Geometry check sheet. Reference: the model listing, model coordinates, mm. Coordinates: 2 decimals unless noted, no trailing zeros. Write each loop counter-clockwise with the first axis right and the second up, starting at its lowest first coordinate (ties: lowest second). Pieces come first, ordered by that corner, then holes. Notation, with made-up numbers: M 13,-21.75 L 35,-21.75 A12 cw 35,-8.75 Z; hole C 80.25,-15.75 d4. An arc over 180 degrees is marked long. Answer as a JSON object with one key per item and string values. Group by question number.
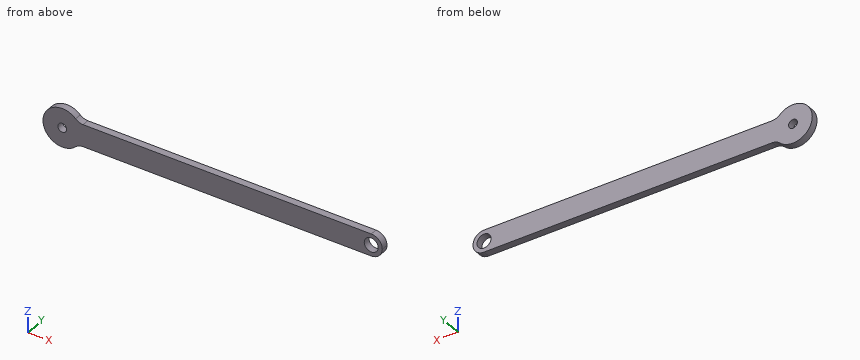
```python
from build123d import *

# Parameters (mm, degrees)
SKETCH1_W           = 300
SKETCH1_H           = 20
BOSS_EXTRUDE1_DEPTH = 6.35
SKETCH2_R           = 6.35
CUT_EXTRUDE1_DEPTH  = 6.35
CONG_1_R            = 10
SKETCH3_R           = 17.5
SKETCH3_R_2         = 4
BOSS_EXTRUDE2_DEPTH = 6.35
FILLET2_R           = 10


with BuildPart() as part:
    # Sketch1 → Boss-Extrude1 (new body)
    with BuildSketch(Plane(origin=(0, 0, 0), x_dir=(1, 0, 0), z_dir=(0, 1, 0))):
        Rectangle(SKETCH1_W, SKETCH1_H)
    extrude(amount=BOSS_EXTRUDE1_DEPTH)

    # Sketch2 → Cut-Extrude1 (cut)
    with BuildSketch(Plane(origin=(0, 0, 0), x_dir=(-1, 0, 0), z_dir=(0, -1, 0))):
        with Locations(Location((140, 0, 0), (0, 0, 90))):
            Circle(SKETCH2_R)
    cut_extrude1 = extrude(amount=-CUT_EXTRUDE1_DEPTH, mode=Mode.SUBTRACT)

    # Mirror1: Cut-Extrude1 across plane
    add(cut_extrude1.mirror(Plane(origin=(0, 0, 0), x_dir=(0, 0, 1), z_dir=(1, 0, 0))), mode=Mode.SUBTRACT)

    # Congé1
    cong_1_edges = [part.edges().sort_by_distance(p)[0] for p in [
        (-150, 3.175, -10),
        (-150, 3.175, 10),
        (150, 3.175, -10),
        (150, 3.175, 10),
    ]]
    fillet(cong_1_edges, radius=CONG_1_R - 0.0001)  # a hair under: the kernel refuses the full size

    # Sketch3 → Boss-Extrude2 (add)
    with BuildSketch(Plane(origin=(0, 6.35, 0), x_dir=(1, 0, 0), z_dir=(0, 1, 0))):
        with Locations((-140, 0)):
            Circle(SKETCH3_R)
        with Locations(Location((-140, 0, 0), (0, 0, 270))):
            Circle(SKETCH3_R_2, mode=Mode.SUBTRACT)
    extrude(amount=-BOSS_EXTRUDE2_DEPTH)

    # Fillet2
    fillet2_edges = [part.edges().sort_by_distance(p)[0] for p in [
        (-125.638593384, 3.175, 10),
        (-125.638593384, 3.175, -10),
    ]]
    fillet(fillet2_edges, radius=FILLET2_R)


solid = part.part
```
1) Go/stop test with flat-tipped pins: pin 1 Ø3 at (y, z) = (4.5, -5.5) entering from -X; pin 2 Ø2 at (x, y) = (45, 3.5) entering from +Z; pin 3 Ø3 at (x, y) = (115, 3) entering from -Z. Record where each tip stops, or that it passes through.
2) Section check B-B (y = 2). State how many separate pieces and enclosed holes the cut face has, then the cut area to 3 significant figures.
3) Section check A-A (x = -140). Record the cut outline in (y, z).
4) Material ranges on probe 1 along X at (y, z) = (3, 0); probe 2 along X at (y, z) = (1.25, -1); probe 3 along Z at (x, y) = (140, 2.25), recorded low to high. Write a range as [from, to].
5) Section check C-C (x = 128.5). Record the cut outline in (y, z).
Entries:
{
 "1": {"pin 1": "x = -157.04", "pin 2": "z = 10", "pin 3": "z = -10"},
 "2": {"separate pieces": "1", "enclosed holes": "2", "area": "6,220 mm^2"},
 "3": {"outline": "M 0,-17.5 L 6.35,-17.5 L 6.35,-4 L 0,-4 Z; M 0,4 L 6.35,4 L 6.35,17.5 L 0,17.5 Z"},
 "4": {"probe 1": "[-157.5, -144], [-136, 133.65], [146.35, 150]", "probe 2": "[-157.47, -143.87], [-136.13, 133.73], [146.27, 149.95]", "probe 3": "[-10, -6.35], [6.35, 10]"},
 "5": {"outline": "M 0,-10 L 6.35,-10 L 6.35,10 L 0,10 Z"}
}
